The listing builds one solid part. Answer for the finished solid, in the listing's coordinates (mm). A direction names the side the tool comes from. Round coordinates to 2 decimals unless told otherwise and drop trailing zeros. Loops run counter-clockwise (first coordinate to the right, second up) from the corner with the lowest first, then second, coordinate; pieces in that order, holes last. Notation, with made-up numbers: M 38.25,30.5 L 93.25,30.5 A31 ccw 93.25,67.5 Z; hole C 73.5,88 d2. An arc over 180 degrees is marked long. Put each result on its own line as item: value. Start each with the question number.
(1) Section C-C, the plane z = 26.5 is taken. Determine the outline of the cut face in (x, y), then the cut area to 3 significant figures.
(2) Section B-B, the plane x = 0 is taken. Determine the outline of the cut face in (y, z).
(3) A flat-ended cylindrical pin translates along its axis: P1, Ø3, axis at x = -1.5, z = -19, coming from the -Y side. Find the tip coordinate at first contact, or state that the pin passes through.
(4) Determine the mould class of faces 1 (the face through (0, 19, 5.2)), 2 (the face through (-15, 10, 0)), 3 (the face through (-0.9, 13.17, -22.45)) for opening direction X: released by +X, released by -X, zero draft, split by the parting line, or undercut.
(5) Straight lines are drawn through the part: line 1 (Z direction, x = 0, y = 11.25); line 2 (Z direction, x = 6.75, y = 17.5); line 3 (X direction, y = 16, z = 26.5). For each, find the intervals that lie inside material, in ascending order.
(6) Section D-D, the plane y = 6.75 is taken. Determine the outline of the cut face in (x, z), then the cut area to 3 significant figures.
(7) Section A-A, the plane y = 22 is taken. Determine the outline of the cut face in (x, z), then the cut area to 3 significant figures.
(8) Which of the six approach directions +Z, -Z, +X, -X, +Y, -Y give full straight-line access (tool end or side, diameter ignored) to faces 4 (the face through (0, 12.3, 0)), 5 (the face through (0, 25, 20))?
```python
from build123d import *

# Parameters (mm, degrees)
SKETCH1_W             = 30
SKETCH1_H             = 70
BOSS_EXTRUDE1_DEPTH   = 25
SKETCH2_W             = 30
SKETCH2_H             = 10.4
CUT_EXTRUDE1_DEPTH    = 12.7
SKETCH3_R             = 4.15
CUT_EXTRUDE2_DEPTH    = 26
CHAMFER1_SIZE         = 1
CHAMFER1_SIZE2        = 1.191753593
CHAMFER1_PART_2_SIZE  = 1
CHAMFER1_PART_2_SIZE2 = 1.191753593


with BuildPart() as part:
    # Sketch1 → Boss-Extrude1 (new body)
    with BuildSketch(Plane(origin=(0, 0, 0), x_dir=(1, 0, 0), z_dir=(0, 1, 0))):
        Rectangle(SKETCH1_W, SKETCH1_H)
    extrude(amount=BOSS_EXTRUDE1_DEPTH)

    # Sketch2 → Cut-Extrude1 (cut)
    with BuildSketch(Plane(origin=(0, 25, 0), x_dir=(1, 0, 0), z_dir=(0, 1, 0))):
        Rectangle(SKETCH2_W, SKETCH2_H)
    extrude(amount=-CUT_EXTRUDE1_DEPTH, mode=Mode.SUBTRACT)

    # Sketch3 → Cut-Extrude2 (cut, through all)
    with BuildSketch(Plane(origin=(0, 25, 0), x_dir=(1, 0, 0), z_dir=(0, 1, 0))):
        with Locations((0, 26.5)):
            Circle(SKETCH3_R)
        with Locations((0, -26.5)):
            Circle(SKETCH3_R)
    extrude(amount=-CUT_EXTRUDE2_DEPTH, mode=Mode.SUBTRACT)

    # Chamfer1
    chamfer1_edges = [part.edges().sort_by_distance(p)[0] for p in [
        (-4.15, 0, -26.5),
    ]]
    chamfer1_side = [part.faces().sort_by_distance(p)[0] for p in [
        (-4.15, 12.5, -26.5),
    ]]
    chamfer(chamfer1_edges, length=CHAMFER1_SIZE, length2=CHAMFER1_SIZE2, reference=chamfer1_side[0])

    # Chamfer1 part 2
    chamfer1_part_2_edges = [part.edges().sort_by_distance(p)[0] for p in [
        (-4.15, 0, 26.5),
    ]]
    chamfer1_part_2_side = [part.faces().sort_by_distance(p)[0] for p in [
        (-4.15, 12.5, 26.5),
    ]]
    chamfer(chamfer1_part_2_edges, length=CHAMFER1_PART_2_SIZE, length2=CHAMFER1_PART_2_SIZE2, reference=chamfer1_part_2_side[0])


solid = part.part
```
Recorded:
1. outline: M -15,0 L -5.34,0 L -4.15,1 L -4.15,25 L -15,25 Z; M 4.15,1 L 5.34,0 L 15,0 L 15,25 L 4.15,25 Z
1. area: 541 mm²
2. outline: M 0,-35 L 25,-35 L 25,-30.65 L 1,-30.65 L 0,-31.84 Z; M 0,-21.16 L 1,-22.35 L 25,-22.35 L 25,-5.2 L 12.3,-5.2 L 12.3,5.2 L 25,5.2 L 25,22.35 L 1,22.35 L 0,21.16 Z; M 0,31.84 L 1,30.65 L 25,30.65 L 25,35 L 0,35 Z
3. P1: stops at y = 0
4. face 1: zero draft
4. face 2: released by -X
4. face 3: undercut
5. line 1: z = -35 to -30.65, -22.35 to 22.35, 30.65 to 35
5. line 2: z = -35 to -5.2, 5.2 to 35
5. line 3: x = -15 to -4.15, 4.15 to 15
6. outline: M -15,-35 L 15,-35 L 15,35 L -15,35 Z; hole C 0,-26.5 d8.3; hole C 0,26.5 d8.3
6. area: 1,990 mm²
7. outline: M -15,-35 L 15,-35 L 15,-5.2 L -15,-5.2 Z; M -15,5.2 L 15,5.2 L 15,35 L -15,35 Z; hole C 0,-26.5 d8.3; hole C 0,26.5 d8.3
7. area: 1,680 mm²
8. face 4: +X, -X, +Y
8. face 5: +Z, -Z, +X, -X, +Y
